from build123d import *

# Parameters (mm, degrees)
ESQUISSE1_R        = 2
ESQUISSE1_R_2      = 1.5
BOSS_EXTRU_1_DEPTH = 3


with BuildPart() as part:
    # Esquisse1 → Boss.-Extru.1 (new body)
    with BuildSketch(Plane.XY):
        Polygon((0, 50), (-100, 50), (-100, 0), (-61.381557247, 0), (-61.381557247, -45.5212086), (-25, -45.5212086), (-25, -80), (25, -80), (25, -45.5212086), (61.381557247, -45.5212086), (61.381557247, 0), (100, 0), (100, 50), align=None)
        with Locations((0, 20)):
            Circle(ESQUISSE1_R, mode=Mode.SUBTRACT)
        with Locations((0, -20)):
            Circle(ESQUISSE1_R, mode=Mode.SUBTRACT)
        with Locations((0, 40)):
            Circle(ESQUISSE1_R, mode=Mode.SUBTRACT)
        with Locations((-20, -55)):
            Circle(ESQUISSE1_R_2, mode=Mode.SUBTRACT)
        with Locations((20, -55)):
            Circle(ESQUISSE1_R_2, mode=Mode.SUBTRACT)
        with Locations((20, -75)):
            Circle(ESQUISSE1_R_2, mode=Mode.SUBTRACT)
        with Locations((-20, -75)):
            Circle(ESQUISSE1_R_2, mode=Mode.SUBTRACT)
        with Locations((-95, 45)):
            Circle(ESQUISSE1_R_2, mode=Mode.SUBTRACT)
        with Locations((-75, 45)):
            Circle(ESQUISSE1_R_2, mode=Mode.SUBTRACT)
        with Locations((-75, 5)):
            Circle(ESQUISSE1_R_2, mode=Mode.SUBTRACT)
        with Locations((-95, 5)):
            Circle(ESQUISSE1_R_2, mode=Mode.SUBTRACT)
        with Locations((75, 5)):
            Circle(ESQUISSE1_R_2, mode=Mode.SUBTRACT)
        with Locations((95, 5)):
            Circle(ESQUISSE1_R_2, mode=Mode.SUBTRACT)
        with Locations((75, 45)):
            Circle(ESQUISSE1_R_2, mode=Mode.SUBTRACT)
        with Locations((95, 45)):
            Circle(ESQUISSE1_R_2, mode=Mode.SUBTRACT)
        with Locations((56.381557247, -40.5212086)):
            Circle(ESQUISSE1_R, mode=Mode.SUBTRACT)
        with Locations((-56.381557247, -40.5212086)):
            Circle(ESQUISSE1_R, mode=Mode.SUBTRACT)
    extrude(amount=BOSS_EXTRU_1_DEPTH)


solid = part.part
Design review of the part built by this model. Coordinates are the model's own, in mm. Give positions to 0.01 mm unless a question says otherwise; leave off trailing zeros. Write each loop counter-clockwise with the first axis right and the second up, starting at its lowest first coordinate (ties: lowest second). Pieces come first, ordered by that corner, then holes. Notation, with made-up numbers: M 33.5,42.5 L 42.5,42.5 A23 ccw 42.5,50.5 Z; hole C -6.5,24.5 d7. An arc over 180 degrees is marked long. Return JSON: item names as keys, results as strings. Group by question number.
Item 1: Wall thickness on line 1 along Y through (x, z) = (0, 1.05); line 2 along Y through (x, z) = (-20, 1); line 3 along Y through (x, z) = (75, 2.05): over which ranges is each line inside the solid? List them lowest first.
Item 2: Take a section at D-D (x = -47.5). Give the boundary of the cut face in (y, z), plus the area to 3 significant figures.
Item 3: Take a section at A-A (x = 0). Give the boundary of the cut face in (y, z), plus the area to 3 significant figures.
Item 4: Take a section at B-B (y = -20). Give the boundary of the cut face in (x, z), plus the area to 3 significant figures.
Item 5: Clearance check with flat-ended pins moving along their axes: pin 1 Ø1.5 at (y, z) = (-63, 1) entering from +X; pin 2 Ø1.5 at (x, z) = (-44.5, 1.5) entering from -Y; pin 3 Ø0.9 at (x, z) = (-82, 2) entering from -Y. State where each tip first meets the part, or that it passes through.
Item 6: Take a section at C-C (z = 0.8). Count the separate pieces of the cut face and the enclosed holes in it, plus the area to 3 significant figures.
Item 7: The part is to be moulded in two halves that separate along Y. For faces 1 (the cylindrical face through (0, 38, 1)), 2 (the flat face through (-1, 0, 3)), 3 (the cylindrical face through (-54.474, -39.92, 1.479)), say which applies: pulls with the +Y half, pulls with the -Y half, needs draft (parallel to the pull), parting line crosses it, or undercut.
Return value:
{
 "1": {"line 1": "y = -80 to -22, -18 to 18, 22 to 38, 42 to 50", "line 2": "y = -80 to -76.5, -73.5 to -56.5, -53.5 to 50", "line 3": "y = 0 to 3.5, 6.5 to 43.5, 46.5 to 50"},
 "2": {"outline": "M -45.52,0 L 50,0 L 50,3 L -45.52,3 Z", "area": "287 mm2"},
 "3": {"outline": "M -80,0 L -22,0 L -22,3 L -80,3 Z; M -18,0 L 18,0 L 18,3 L -18,3 Z; M 22,0 L 38,0 L 38,3 L 22,3 Z; M 42,0 L 50,0 L 50,3 L 42,3 Z", "area": "354 mm2"},
 "4": {"outline": "M -61.38,0 L -2,0 L -2,3 L -61.38,3 Z; M 2,0 L 61.38,0 L 61.38,3 L 2,3 Z", "area": "356 mm2"},
 "5": {"pin 1": "stops at x = 25", "pin 2": "stops at y = -45.52", "pin 3": "stops at y = 0"},
 "6": {"separate pieces": "1", "enclosed holes": "17", "area": "17,200 mm2"},
 "7": {"face 1": "undercut", "face 2": "needs draft", "face 3": "undercut"}
}
